from build123d import *

# Parameters (mm, degrees)
SKETCH_1_R          = 4.1
SKETCH_1_R_2        = 2.5
EXTRUDE_1_DEPTH     = 10
CUT_EXTRUDE_3_REACH = 92.692
CUT_EXTRUDE_START   = 3
CUT_EXTRUDE_4_DEPTH = 3
SKETCH_7_R          = 5.1
CUT_EXTRUDE_5_DEPTH = 5
SKETCH_8_R          = 4
CUT_EXTRUDE_6_DEPTH = 2.5
SKETCH_9_R          = 1.5
CUT_EXTRUDE_7_DEPTH = 91.691785736
SKETCH_10_W         = 10.2
SKETCH_10_H         = 10.2
CUT_EXTRUDE_8_DEPTH = 5


with BuildPart() as part:
    # ｽｹｯﾁ1 → ﾎﾞｽ - 押し出し1 (new body)
    with BuildSketch(Plane(origin=(0, 0, 0), x_dir=(1, 0, 0), z_dir=(0, 1, 0))):
        with BuildLine():
            Line((-65, -50), (65, -50))
            ThreePointArc((65, -50), (72.071067812, -47.071067812), (75, -40))
            Line((75, -40), (75, 40))
            ThreePointArc((75, 40), (72.071067812, 47.071067812), (65, 50))
            Line((65, 50), (-65, 50))
            ThreePointArc((-65, 50), (-72.071067812, 47.071067812), (-75, 40))
            Line((-75, 40), (-75, -40))
            ThreePointArc((-75, -40), (-72.071067812, -47.071067812), (-65, -50))
        make_face()
        with Locations(Location((55, 0, 0), (0, 0, 270))):
            Circle(SKETCH_1_R, mode=Mode.SUBTRACT)
        with Locations(Location((43, 12, 0), (0, 0, 270))):
            Circle(SKETCH_1_R_2, mode=Mode.SUBTRACT)
        with Locations(Location((67, 12, 0), (0, 0, 270))):
            Circle(SKETCH_1_R_2, mode=Mode.SUBTRACT)
        with Locations(Location((67, -12, 0), (0, 0, 270))):
            Circle(SKETCH_1_R_2, mode=Mode.SUBTRACT)
        with Locations(Location((43, -12, 0), (0, 0, 270))):
            Circle(SKETCH_1_R_2, mode=Mode.SUBTRACT)
        with Locations(Location((-55, 0, 0), (0, 0, 270))):
            Circle(SKETCH_1_R, mode=Mode.SUBTRACT)
    extrude(amount=EXTRUDE_1_DEPTH)

    # ｽｹｯﾁ5 → ｶｯﾄ - 押し出し3 (cut, up to next)
    with BuildSketch(Plane(origin=(0, 10, 0), x_dir=(1, 0, 0), z_dir=(0, 1, 0)), mode=Mode.PRIVATE) as cut_extrude_3_sk1:
        with BuildLine():
            Line((-18.5, 28.2), (-17.5, 28.2))
            ThreePointArc((-17.5, 28.2), (10.7, 0), (-17.5, -28.2))
            Line((-17.5, -28.2), (-18.5, -28.2))
            ThreePointArc((-18.5, -28.2), (-46.7, 0), (-18.5, 28.2))
        make_face()
    cut_extrude_3_tool1 = extrude(cut_extrude_3_sk1.sketch, amount=-CUT_EXTRUDE_3_REACH, mode=Mode.PRIVATE) & part.part
    # ｽｹｯﾁ5 → ｶｯﾄ - 押し出し3 (cut, up to next)
    with BuildSketch(Plane(origin=(0, 10, 0), x_dir=(1, 0, 0), z_dir=(0, 1, 0)), mode=Mode.PRIVATE) as cut_extrude_3_sk2:
        with BuildLine():
            Line((-18.5, 41.6), (-17.5, 41.6))
            ThreePointArc((-17.5, 41.6), (-15.9, 40), (-17.5, 38.4))
            Line((-17.5, 38.4), (-18.5, 38.4))
            ThreePointArc((-18.5, 38.4), (-20.1, 40), (-18.5, 41.6))
        make_face()
    cut_extrude_3_tool2 = extrude(cut_extrude_3_sk2.sketch, amount=-CUT_EXTRUDE_3_REACH, mode=Mode.PRIVATE) & part.part
    # ｽｹｯﾁ5 → ｶｯﾄ - 押し出し3 (cut, up to next)
    with BuildSketch(Plane(origin=(0, 10, 0), x_dir=(1, 0, 0), z_dir=(0, 1, 0)), mode=Mode.PRIVATE) as cut_extrude_3_sk3:
        with BuildLine():
            Line((-18.5, -38.4), (-17.5, -38.4))
            ThreePointArc((-17.5, -38.4), (-15.9, -40), (-17.5, -41.6))
            Line((-17.5, -41.6), (-18.5, -41.6))
            ThreePointArc((-18.5, -41.6), (-20.1, -40), (-18.5, -38.4))
        make_face()
    cut_extrude_3_tool3 = extrude(cut_extrude_3_sk3.sketch, amount=-CUT_EXTRUDE_3_REACH, mode=Mode.PRIVATE) & part.part
    add(cut_extrude_3_tool1.solids().sort_by_distance((-18, 10, 0))[0], mode=Mode.SUBTRACT)
    add(cut_extrude_3_tool2.solids().sort_by_distance((-18, 10, -40))[0], mode=Mode.SUBTRACT)
    add(cut_extrude_3_tool3.solids().sort_by_distance((-18, 10, 40))[0], mode=Mode.SUBTRACT)

    # ｽｹｯﾁ6 → ｶｯﾄ - 押し出し4 (cut)
    with BuildSketch(Plane(origin=(0, 0, 0), x_dir=(1, 0, 0), z_dir=(0, 1, 0)).offset(CUT_EXTRUDE_START)):
        with BuildLine():
            Line((-18.5, 45.2), (-17.5, 45.2))
            ThreePointArc((-17.5, 45.2), (-13.823044738, 43.676955262), (-12.3, 40))
            Line((-12.3, 40), (-12.3, 27.716421125))
            ThreePointArc((-12.3, 27.716421125), (10.7, 0), (-12.3, -27.716421125))
            Line((-12.3, -27.716421125), (-12.3, -40))
            ThreePointArc((-12.3, -40), (-13.823044738, -43.676955262), (-17.5, -45.2))
            Line((-17.5, -45.2), (-18.5, -45.2))
            ThreePointArc((-18.5, -45.2), (-22.176955262, -43.676955262), (-23.7, -40))
            Line((-23.7, -40), (-23.7, -27.716421125))
            ThreePointArc((-23.7, -27.716421125), (-46.7, 0), (-23.7, 27.716421125))
            Line((-23.7, 27.716421125), (-23.7, 40))
            ThreePointArc((-23.7, 40), (-22.176955262, 43.676955262), (-18.5, 45.2))
        make_face()
    extrude(amount=-CUT_EXTRUDE_4_DEPTH, mode=Mode.SUBTRACT)

    # ｽｹｯﾁ7 → ｶｯﾄ - 押し出し5 (cut)
    with BuildSketch(Plane.XZ):
        with Locations(Location((20, 0, 0), (0, 0, 270))):
            Circle(SKETCH_7_R)
    extrude(amount=-CUT_EXTRUDE_5_DEPTH, mode=Mode.SUBTRACT)

    # ｽｹｯﾁ8 → ｶｯﾄ - 押し出し6 (cut)
    with BuildSketch(Plane(origin=(0, 10, 0), x_dir=(1, 0, 0), z_dir=(0, 1, 0))):
        with Locations(Location((43, 12, 0), (0, 0, 270))):
            Circle(SKETCH_8_R)
        with Locations(Location((67, 12, 0), (0, 0, 270))):
            Circle(SKETCH_8_R)
        with Locations(Location((43, -12, 0), (0, 0, 270))):
            Circle(SKETCH_8_R)
        with Locations(Location((67, -12, 0), (0, 0, 270))):
            Circle(SKETCH_8_R)
    extrude(amount=-CUT_EXTRUDE_6_DEPTH, mode=Mode.SUBTRACT)

    # ｽｹｯﾁ9 → ｶｯﾄ - 押し出し7 (cut, through all)
    with BuildSketch(Plane(origin=(0, 10, 0), x_dir=(1, 0, 0), z_dir=(0, 1, 0))):
        with Locations(Location((-60, 35, 0), (0, 0, 270))):
            Circle(SKETCH_9_R)
        with Locations(Location((-60, -35, 0), (0, 0, 270))):
            Circle(SKETCH_9_R)
    extrude(amount=-CUT_EXTRUDE_7_DEPTH, mode=Mode.SUBTRACT)

    # ｽｹｯﾁ10 → ｶｯﾄ - 押し出し8 (cut)
    with BuildSketch(Plane(origin=(0, 10, 0), x_dir=(1, 0, 0), z_dir=(0, 1, 0))):
        with Locations((-60, 35)):
            Rectangle(SKETCH_10_W, SKETCH_10_H)
        with Locations((-60, -35)):
            Rectangle(SKETCH_10_W, SKETCH_10_H)
    extrude(amount=-CUT_EXTRUDE_8_DEPTH, mode=Mode.SUBTRACT)


solid = part.part
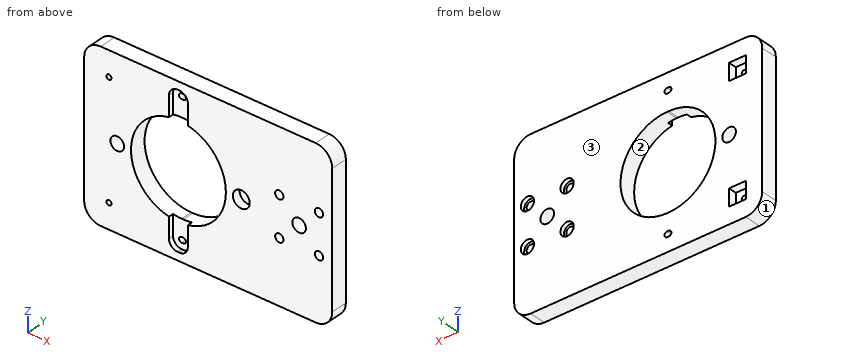
Work out the finished part from the listing and answer in its coordinate system (mm). Face numbers are marked on the shaded views. Coordinates: 2 decimals unless noted, no trailing zeros. Write each loop counter-clockwise with the first axis right and the second up, starting at its lowest first coordinate (ties: lowest second). Pieces come first, ordered by that corner, then holes. Notation, with made-up numbers: (-34, 39.25) - (-28, 39.25) arc R20 ccw to (-28, 54.25) - close; hole circle Ø1 at (57.5, 30.25). An arc over 180 degrees is marked (long way). One line per question, with ' | ' between items.
1) Find section C-C, the plane z = 18. Determine the outline of the cut face in (x, y), and give its area (3 significant figures).
Checks:
outline: (-75, 0) - (-40.21, 0) - (-40.21, 10) - (-75, 10) - close; (4.21, 0) - (75, 0) - (75, 10) - (4.21, 10) - close | area: 1,060 mm2
2) Flat-ended cylindrical pins translate along their axes: P1, Ø13.5, axis at x = 20, z = 0, coming from the -Y side; P2, Ø3, axis at x = -58, z = -35.5, coming from the +Y side; P3, Ø6.5, axis at x = 66.5, z = 11.5, coming from the +Y side. Find the tip coordinate at first contact, or state that the pin passes through.
Checks:
P1: y = 0 | P2: y = 5 | P3: y = 7.5
3) Consider probe 1 along X at (y, z) = (3.55, 0); probe 2 along X at (y, z) = (7, 0); probe 3 along Z at (x, y) = (43, 5.25). Determine where each line is inside the solid, lowest interval first. Write a range as [from, to].
Checks:
probe 1: [-75, -59.1], [-50.9, -46.7], [10.7, 14.9], [25.1, 50.9], [59.1, 75] | probe 2: [-75, -59.1], [-50.9, -46.7], [10.7, 50.9], [59.1, 75] | probe 3: [-50, -14.5], [-9.5, 9.5], [14.5, 50]
4) Find section B-B, the plane z = -12.5. Determine the outline of the cut face in (x, y), and give its area (3 significant figures).
Checks:
outline: (-75, 0) - (-43.78, 0) - (-43.78, 10) - (-75, 10) - close; (7.78, 0) - (40.55, 0) - (40.55, 7.5) - (39.03, 7.5) - (39.03, 10) - (7.78, 10) - close; (45.45, 0) - (64.55, 0) - (64.55, 7.5) - (63.03, 7.5) - (63.03, 10) - (46.97, 10) - (46.97, 7.5) - (45.45, 7.5) - close; (69.45, 0) - (75, 0) - (75, 10) - (70.97, 10) - (70.97, 7.5) - (69.45, 7.5) - close | area: 871 mm2
5) Find section A-A, the plane z = 35. Determine the outline of the cut face in (x, y), and give its area (3 significant figures).
Checks:
outline: (-75, 0) - (-61.5, 0) - (-61.5, 5) - (-65.1, 5) - (-65.1, 10) - (-75, 10) - close; (-58.5, 0) - (-23.7, 0) - (-23.7, 3) - (-12.3, 3) - (-12.3, 0) - (75, 0) - (75, 10) - (-54.9, 10) - (-54.9, 5) - (-58.5, 5) - close | area: 1,400 mm2
6) The mould has two halves that part along X. Classify the marked faces 1, 2 and 3: +X half, -X half, draft (parallel to the pull), parting line (faces both ways), or undercut.
Checks:
face 1: -X half | face 2: undercut | face 3: draft
